Check sheet for the modelled part. Datum: model origin and axes. Units: mm. Face numbers are marked on the shaded views. A direction names the side the tool comes from. Give positions to 0.01 mm unless a question says otherwise; leave off trailing zeros. Write each loop counter-clockwise with the first axis right and the second up, starting at its lowest first coordinate (ties: lowest second). Pieces come first, ordered by that corner, then holes. Notation, with made-up numbers: (65.5, 49) -> (69.5, 49) arc R30 ccw to (69.5, 76) -> close; hole circle Ø7 at (-17.75, 82). An arc over 180 degrees is marked (long way). Return JSON: item names as keys, results as strings.
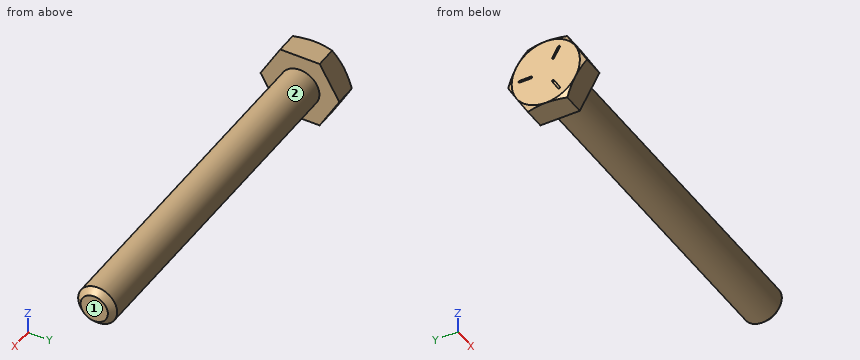
from build123d import *

# Parameters (mm, degrees)
SKETCH5_R           = 3.175
BOSS_EXTRUDE3_DEPTH = 57.15
CHAMFER1_SIZE       = 0.9525
BOSS_EXTRUDE4_DEPTH = 3.96875
SKETCH8_OUTSIDE_W   = 240.984
SKETCH8_OUTSIDE_H   = 242.704
SKETCH8_OUTSIDE_R   = 5.55625
CUT_EXTRUDE3_DEPTH  = 62.11875
CUT_EXTRUDE3_TAPER  = 60
CUT_EXTRUDE4_DEPTH  = 0.254
CIRPATTERN1_COUNT   = 3


with BuildPart() as part:
    # Sketch5 → Boss-Extrude3 (new body)
    with BuildSketch(Plane(origin=(30.559375, 0, 0), x_dir=(0, 0, -1), z_dir=(1, 0, 0))):
        Circle(SKETCH5_R)
    extrude(amount=-BOSS_EXTRUDE3_DEPTH)

    # Chamfer1
    chamfer1_edges = [part.edges().sort_by_distance(p)[0] for p in [
        (30.559375, 0, 3.175),
    ]]
    chamfer(chamfer1_edges, length=CHAMFER1_SIZE)

    # Sketch11 → Revolve1 (revolve)
    with BuildSketch(Plane.XY):
        Polygon((-26.590625, 3.175), (-26.590625, 0), (14.684375, 0), (11.509375, 3.175), align=None)
    revolve(axis=Axis((-26.590625, 0, 0), (1, 0, 0)))

    # Sketch6 → Boss-Extrude4 (add)
    with BuildSketch(Plane.ZY.offset(26.590625)):
        Polygon((5.55625, 3.207902433), (0, 6.415804866), (-5.55625, 3.207902433), (-5.55625, -3.207902433), (0, -6.415804866), (5.55625, -3.207902433), align=None)
    extrude(amount=BOSS_EXTRUDE4_DEPTH)

    # Sketch8 outside → Cut-Extrude3 (cut, through all)
    with BuildSketch(Plane.ZY.offset(30.559375)):
        Rectangle(SKETCH8_OUTSIDE_W, SKETCH8_OUTSIDE_H)
        Circle(SKETCH8_OUTSIDE_R, mode=Mode.SUBTRACT)
    extrude(amount=-CUT_EXTRUDE3_DEPTH, taper=CUT_EXTRUDE3_TAPER, mode=Mode.SUBTRACT)

    # Sketch12 → Cut-Extrude4 (cut)
    with BuildSketch(Plane.ZY.offset(30.559375)):
        with BuildLine():
            Line((0.1666875, 4.2783125), (0.1666875, 2.3891875))
            ThreePointArc((0.1666875, 2.3891875), (0, 2.2225), (-0.1666875, 2.3891875))
            Line((-0.1666875, 2.3891875), (-0.1666875, 4.2783125))
            ThreePointArc((-0.1666875, 4.2783125), (0, 4.445), (0.1666875, 4.2783125))
        make_face()
    cut_extrude4 = extrude(amount=-CUT_EXTRUDE4_DEPTH, mode=Mode.SUBTRACT)

    # CirPattern1: Cut-Extrude4 ×3 about axis
    cirpattern1_axis = Axis((0, 0, 0), (1, 0, 0))
    for i in range(1, CIRPATTERN1_COUNT):
        add(cut_extrude4.rotate(cirpattern1_axis, i * 360 / CIRPATTERN1_COUNT), mode=Mode.SUBTRACT)


solid = part.part
(1) Thickness scan on L1, parallel to X at y = -3, z = -4; L2, parallel to Z at x = 6.5, y = 0.25; L3, parallel to Y at x = -19.5, z = 2.25. Record the ranges inside material, lowest first.
Reply:
{"L1": "-30.56 to -26.59", "L2": "-3.17 to 3.17", "L3": "-2.24 to 2.24"}
(2) Depth check by flat-ended pin: pin 1 Ø1 at (x, z) = (1.5, 3) entering from +Y; pin 2 Ø2 at (x, z) = (19, -3) entering from -Y; pin 3 Ø1.5 at (x, y) = (-16.5, -2.5) entering from -Z. Enter the tip coordinate at first touch or a pass-through.
Reply:
{"pin 1": "y = 1.96", "pin 2": "y = -2.47", "pin 3": "z = -2.65"}
(3) Set-up check for the marked faces 1 and 2: record each of +Z, -Z, +X, -X, +Y, -Y from which the full face is reachable in a straight line by a thin tool's end or side.
Reply:
{"face 1": "+Z, -Z, +X, +Y, -Y", "face 2": "+X"}
(4) Cross-section at A-A on x = 7.5. Enter the section's corners in (y, z) (3 decimals).
Reply:
{"outline": "circle Ø6.35 at (0, 0)"}
